Autodesk Inventor part; units mm, degrees
ref_plane "YZ Plane" through (0, 0, 0) normal (1, 0, 0) x (0, 1, 0)
ref_plane "XZ Plane" through (0, 0, 0) normal (0, 1, 0) x (-1, 0, 0)
ref_plane "XY Plane" through (0, 0, 0) normal (0, 0, 1) x (1, 0, 0)
sketch "Sketch1" plane through (0, 0, 0) normal (0, 0, 1) x (1, 0, 0)
  line L0 (0, 0) -> (30, 0)
  line L1 (30, 0) -> (30, 30)
  line L2 (30, 30) -> (0, 30)
  line L3 (0, 30) -> (0, 0)
  line L4 (30, 30) -> (3, 30)
  line L5 (3, 30) -> (3, 3)
  line L6 (3, 3) -> (30, 3)
  line L7 (30, 3) -> (30, 30)
  point P0 (3, 30)
  dimension "d0" = 30
  dimension "d1" = 30
  dimension "d4" = 27
  dimension "d5" = 27
extrude "Extrusion1" add sketch "Sketch1" along normal blind 320 contours L3 L2 L5 L6 L1 L0
properties part number "frame side" material "Aluminum 6061"
The model under review builds one solid part; all positions refer to its coordinate system, in mm. A direction names the side the tool comes from. Give positions to 0.01 mm unless a question says otherwise; leave off trailing zeros. Order: outer loops, then holes, each group sorted by start corner. A loop starts at its lowest first (then second) coordinate and runs counter-clockwise, first axis right, second up. Notation, with made-up numbers: M 35.5,55 L 70.5,55 A33 ccw 70.5,89 Z; hole C 29,-18.75 d4. An arc over 180 degrees is marked long. Answer in a Markdown table with one row per item. Add a question column.
1. To check wall thickness, follow line 1 along X through (y, z) = (3.75, 141). State the ranges of the line that lie inside material, in increasing order.
2. Add section A-A on z = 103. State the section outline as (x, y) points, plus the area to 3 significant figures.
3. Add section B-B on y = 10.25. State the section outline as (x, z) points, plus the area to 3 significant figures.
4. For pin 1 Ø10 at (y, z) = (8.5, 183) entering from +X; pin 2 Ø8 at (x, z) = (15, 164.5) entering from +Y, all flat-tipped, find the tip position at first contact; note any pin that passes through.
5. Machinability: for faces 1 (the flat face through (16, 3, 158)), 2 (the flat face through (8.3, 2.8, 0)), which of the approach directions +Z, -Z, +X, -X, +Y, -Y give a long, thin tool a straight path to every point of the face, cutting with its end or side? Answer none if there is none.
The answers:
| question | item | result |
|---|---|---|
| 1 | line 1 | 0 to 3 |
| 2 | outline | M 0,0 L 30,0 L 30,3 L 3,3 L 3,30 L 0,30 Z |
| 2 | area | 171 mm2 |
| 3 | outline | M 0,0 L 3,0 L 3,320 L 0,320 Z |
| 3 | area | 960 mm2 |
| 4 | pin 1 | x = 3 |
| 4 | pin 2 | y = 3 |
| 5 | face 1 | +Z, -Z, +X, +Y |
| 5 | face 2 | -Z, +X, -X, +Y, -Y |
